For this review, take the finished solid that the model builds, in its own axes (mm). A direction names the side the tool comes from. Coordinates: 2 decimals unless noted, no trailing zeros. Order: outer loops, then holes, each group sorted by start corner. A loop starts at its lowest first (then second) coordinate and runs counter-clockwise, first axis right, second up.
from build123d import *

# Parameters (mm, degrees)
SKETCH1_W           = 152.4
SKETCH1_H           = 177.8
BOSS_EXTRUDE1_DEPTH = 1
SKETCH15_W          = 152.4
SKETCH15_H          = 2
EXTRUDE_THIN1_DEPTH = 127
SKETCH16_W          = 152.4
SKETCH16_H          = 1
EXTRUDE_THIN2_DEPTH = 12.7
SKETCH17_W          = 152.4
SKETCH17_H          = 1
EXTRUDE_THIN3_DEPTH = 12.7
SKETCH18_W          = 152.4
SKETCH18_H          = 1
EXTRUDE_THIN4_DEPTH = 173.8


with BuildPart() as part:
    # Sketch1 → Boss-Extrude1 (new body)
    with BuildSketch(Plane(origin=(0, 0, 0), x_dir=(1, 0, 0), z_dir=(0, 1, 0))):
        Rectangle(SKETCH1_W, SKETCH1_H)
    extrude(amount=BOSS_EXTRUDE1_DEPTH)

    # Sketch15 → Extrude-Thin1 (add)
    with BuildSketch(Plane(origin=(0, 1, 0), x_dir=(1, 0, 0), z_dir=(0, 1, 0))):
        with Locations((0, -87.9)):
            Rectangle(SKETCH15_W, SKETCH15_H)
        with Locations((0, 87.9)):
            Rectangle(SKETCH15_W, SKETCH15_H)
    extrude(amount=EXTRUDE_THIN1_DEPTH)

    # Sketch16 → Extrude-Thin2 (add)
    with BuildSketch(Plane(origin=(0, 0, 86.9), x_dir=(-1, 0, 0), z_dir=(0, 0, -1))):
        with Locations((0, 25.9)):
            Rectangle(SKETCH16_W, SKETCH16_H)
        with Locations((0, 51.3)):
            Rectangle(SKETCH16_W, SKETCH16_H)
        with Locations((0, 76.7)):
            Rectangle(SKETCH16_W, SKETCH16_H)
        with Locations((0, 102.1)):
            Rectangle(SKETCH16_W, SKETCH16_H)
    extrude(amount=EXTRUDE_THIN2_DEPTH)

    # Sketch17 → Extrude-Thin3 (add)
    with BuildSketch(Plane.XY.offset(-86.9)):
        with Locations((0, 26.9)):
            Rectangle(SKETCH17_W, SKETCH17_H)
        with Locations((0, 52.3)):
            Rectangle(SKETCH17_W, SKETCH17_H)
        with Locations((0, 77.7)):
            Rectangle(SKETCH17_W, SKETCH17_H)
        with Locations((0, 103.1)):
            Rectangle(SKETCH17_W, SKETCH17_H)
    extrude(amount=EXTRUDE_THIN3_DEPTH)

    # Sketch18 → Extrude-Thin4 (add)
    with BuildSketch(Plane(origin=(0, 0, 86.9), x_dir=(-1, 0, 0), z_dir=(0, 0, -1))):
        with Locations((0, 127.5)):
            Rectangle(SKETCH18_W, SKETCH18_H)
    extrude(amount=EXTRUDE_THIN4_DEPTH)


solid = part.part
1. To check wall thickness, follow L1, parallel to Y at x = 68.5, z = 4.5; L2, parallel to Z at x = -50.5, y = 99; L3, parallel to Z at x = -43, y = 52. State the ranges of each line that lie inside material, in increasing order.
Answer below:
L1: y = 0 to 1, 127 to 128
L2: z = -88.9 to -86.9, 86.9 to 88.9
L3: z = -88.9 to -74.2, 86.9 to 88.9
2. Clearance check with a flat-ended pin moving along its axis: pin 1 Ø3 at (x, z) = (-36.5, -43) entering from -Y. State where the tip first meets the part, or that it passes through.
Answer below:
pin 1: stops at y = 0
3. Machinability: for faces 1 (the face through (-1, 0, -1)), 2 (the face through (1, 101.6, 81)), which of the approach directions +Z, -Z, +X, -X, +Y, -Y give a long, thin tool a straight path to every point of the face, cutting with its end or side? Answer none if there is none.
Answer below:
face 1: +Z, -Z, +X, -X, -Y
face 2: +X, -X
4. Take a section at A-A, the plane y = 37. Give the boundary of the cut face in (x, z), plus the area to 3 significant figures.
Answer below:
outline: (-76.2, -88.9) - (76.2, -88.9) - (76.2, -86.9) - (-76.2, -86.9) - close; (-76.2, 86.9) - (76.2, 86.9) - (76.2, 88.9) - (-76.2, 88.9) - close
area: 610 mm2
5. Take a section at B-B, the plane z = 20. Give the boundary of the cut face in (x, y).
Answer below:
outline: (-76.2, 0) - (76.2, 0) - (76.2, 1) - (-76.2, 1) - close; (-76.2, 127) - (76.2, 127) - (76.2, 128) - (-76.2, 128) - close
